Work out the finished part from the listing and answer in its coordinate system (mm). Face numbers are marked on the shaded views. A direction names the side the tool comes from. Coordinates: 2 decimals unless noted, no trailing zeros. Write each loop counter-clockwise with the first axis right and the second up, starting at its lowest first coordinate (ties: lowest second). Pieces come first, ordered by that corner, then holes. Notation, with made-up numbers: (42, -5) - (94, -5) arc R25 cw to (94, 27) - close; hole circle Ø5 at (34.25, -25.75). An arc over 180 degrees is marked (long way). Use one line per item in the form item = value. Start each with the question number.
Item 1: A cutting plane is placed at D-D (x = 15). Write down the section's boundary in (y, z), then the cut area to 3 significant figures.
Item 2: A cutting plane is placed at C-C (x = -1). Write down the section's boundary in (y, z).
Item 3: A cutting plane is placed at B-B (z = 5). Write down the section's boundary in (x, y), then the cut area to 3 significant figures.
Item 4: Consider probe 1 along X at (y, z) = (18, 6.25); probe 2 along Z at (x, y) = (15, 4.75); probe 3 along Y at (x, z) = (2, 5.5). Determine where each line is inside the solid, lowest interval first.
Item 5: For the marked faces 4, 5 and 6, determine the directions among +Z, -Z, +X, -X, +Y, -Y from which every point of the face is accessible in a straight line to the end or side of a thin tool.
Item 6: A cutting plane is placed at A-A (y = 49). Write down the section's boundary in (x, z), then the cut area to 3 significant figures.
Item 7: Determine the mould class of the marked faces 1, 2 and 3 for opening direction Y: released by +Y, released by -Y, zero draft, split by the parting line, or undercut.
Item 8: Given pin 1 (2 mm diameter, centred on x = 15, z = 5, fed in from -Y); pin 2 (3 mm diameter, centred on x = 0.5, z = 5.5, fed in from +Y); pin 3 (6 mm diameter, centred on x = -5, y = 46, fed in from -Z), each flat-ended and moving along its own axis, determine where each tip first touches the part or whether it passes through.
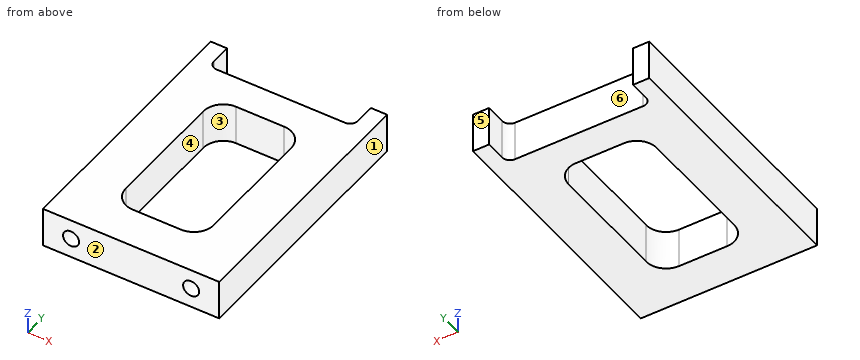
from build123d import *

# Parameters (mm, degrees)
BOSS_EXTRUDE1_DEPTH = 10
SKETCH2_R           = 2
CUT_EXTRUDE1_DEPTH  = 10
FILLET1_R           = 2
SKETCH3_W           = 22
SKETCH3_H           = 40
CUT_EXTRUDE2_DEPTH  = 11
FILLET2_R           = 5


with BuildPart() as part:
    # Sketch1 → Boss-Extrude1 (new body)
    with BuildSketch(Plane.XY):
        Polygon((-22, 0), (22, 0), (22, 65), (18, 65), (18, 58), (-18, 58), (-18, 65), (-22, 65), align=None)
    extrude(amount=BOSS_EXTRUDE1_DEPTH)

    # Sketch2 → Cut-Extrude1 (cut)
    with BuildSketch(Plane.XZ):
        with Locations((15, 5)):
            Circle(SKETCH2_R)
        with Locations((-15, 5)):
            Circle(SKETCH2_R)
    extrude(amount=-CUT_EXTRUDE1_DEPTH, mode=Mode.SUBTRACT)

    # Fillet1
    fillet1_edges = [part.edges().sort_by_distance(p)[0] for p in [
        (-18, 58, 5),
        (18, 58, 5),
    ]]
    fillet(fillet1_edges, radius=FILLET1_R)

    # Sketch3 → Cut-Extrude2 (cut, through all)
    with BuildSketch(Plane(origin=(0, 0, 0), x_dir=(-1, 0, 0), z_dir=(0, 0, -1))):
        with Locations((0, 30)):
            Rectangle(SKETCH3_W, SKETCH3_H)
    extrude(amount=-CUT_EXTRUDE2_DEPTH, mode=Mode.SUBTRACT)

    # Fillet2
    fillet2_edges = [part.edges().sort_by_distance(p)[0] for p in [
        (11, 10, 5),
        (11, 50, 5),
        (-11, 50, 5),
        (-11, 10, 5),
    ]]
    fillet(fillet2_edges, radius=FILLET2_R)


solid = part.part
Answer:
q1.outline = (0, 0) - (58, 0) - (58, 10) - (0, 10) - (0, 7) - (10, 7) - (10, 3) - (0, 3) - close
q1.area = 540 mm²
q2.outline = (0, 0) - (10, 0) - (10, 10) - (0, 10) - close; (50, 0) - (58, 0) - (58, 10) - (50, 10) - close
q3.outline = (-22, 0) - (-17, 0) - (-17, 10) - (-13, 10) - (-13, 0) - (13, 0) - (13, 10) - (17, 10) - (17, 0) - (22, 0) - (22, 65) - (18, 65) - (18, 60) arc R2 cw to (16, 58) - (-16, 58) arc R2 cw to (-18, 60) - (-18, 65) - (-22, 65) - close; hole (-11, 15) arc R5 ccw to (-6, 10) - (6, 10) arc R5 ccw to (11, 15) - (11, 45) arc R5 ccw to (6, 50) - (-6, 50) arc R5 ccw to (-11, 45) - close
q3.area = 1,670 mm²
q4.probe_1 = -22 to -11, 11 to 22
q4.probe_2 = 0 to 3, 7 to 10
q4.probe_3 = 0 to 10, 50 to 58
q5.face_4 = +Z, -Z
q5.face_5 = +Z, -Z, +X, -X, +Y
q5.face_6 = +Z, -Z, +Y
q6.outline = (-22, 0) - (-9, 0) - (-9, 10) - (-22, 10) - close; (9, 0) - (22, 0) - (22, 10) - (9, 10) - close
q6.area = 260 mm²
q7.face_1 = zero draft
q7.face_2 = released by -Y
q7.face_3 = undercut
q8.pin_1 = 10
q8.pin_2 = 58
q8.pin_3 = through
